Here's how the part is built. I have some questions about the finished solid (model axes, mm). A direction names the side the tool comes from. Give positions to 0.01 mm unless a question says otherwise; leave off trailing zeros. Write each loop counter-clockwise with the first axis right and the second up, starting at its lowest first coordinate (ties: lowest second). Pieces come first, ordered by that corner, then holes. Notation, with made-up numbers: M -15,-9 L 29,-9 A31 cw 29,24 Z; hole C -10.75,83 d10. An arc over 180 degrees is marked long. Answer as CSV lines item,"result". Start each with the question number.
Q1. If I drill on line 1 along X through (y, z) = (117, 0); line 2 along Z through (x, y) = (0, 81.5); line 3 along X through (y, z) = (85.5, -45), over which ranges is the centre line in solid material (lowest first)?
Q2. Suppose I cut it at D-D (z = 88). Write out the boundary of the cut face in (x, y) (1 decimal).
Q3. Thinking about a two-plate mould opening in Z: for faces 4 (the cylindrical face through (-4.62, 4.7, 144.39)), 5 (the flat face through (-1, 0, 123)), 6 (the cylindrical face through (122.834, 4.696, -50.878)), which applies, +Z half, -Z half, draft (parallel to the pull), parting line (faces both ways), or undercut?
Q4. Suppose I cut it at B-B (x = 44). Write out the boundary of the cut face in (y, z) (1 decimal).
Q5. Suppose I cut it at A-A (z = 0). Write out the boundary of the cut face in (x, y) (1 decimal).
Q6. Suppose I cut it at C-C (x = 83.5). Write out the boundary of the cut face in (y, z) (1 decimal), then the cut area to 3 significant figures.
Q7. On a 3-axis mill with a long thin cutter (end or side, diameter ignored), from which of +Z, -Z, +X, -X, +Y, -Y can I reach the whole of each face in a straight line? I mean faces 1 (the flat face through (-1, 9.525, 132)), 2 (the cylindrical face through (3.44, 55.567, 121.395)), 3 (the flat face through (-109.22, 43, -64)). Say none if no direction works.
Q8. For pin 1 (1.5 mm diameter, centred on y = 102.5, z = -12, fed in from +X); pin 2 (12 mm diameter, centred on x = 30, z = -86.5, fed in from -Y); pin 3 (5.5 mm diameter, centred on x = 126.13, z = -52.25, fed in from -Y); pin 4 (5 mm diameter, centred on y = 37.5, z = 82, fed in from +X), each with a flat end and sliding along its axis, tell me the tip position at first contact or that it passes through.
```python
from build123d import *

# Parameters (mm, degrees)
SKETCH1_R                   = 144.4625
BOSS_EXTRUDE1_DEPTH         = 9.525
F_1_4_CLEARANCE_HOLE1_D     = 7.14248
SKETCH4_R                   = 127.79375
SKETCH4_R_2                 = 121.44375
BOSS_EXTRUDE2_DEPTH         = 112.7125
BOSS_EXTRUDE3_START         = -9.525
SKETCH5_R                   = 121.44375
BOSS_EXTRUDE3_DEPTH         = 9.525
CUT_EXTRUDE1_REACH          = 240.077
SKETCH6_R                   = 121.44375
CUT_EXTRUDE2_REACH          = 240.077
SKETCH7_R                   = 51.59375
SKETCH10_W                  = 218.44
SKETCH10_H                  = 91.362820019
CUT_EXTRUDE3_DEPTH          = 112.7125
TAP_DRILL_FOR_1_4_20_TAP1_D = 5.1054


with BuildPart() as part:
    # Sketch1 → Boss-Extrude1 (new body)
    with BuildSketch(Plane(origin=(0, 0, 0), x_dir=(1, 0, 0), z_dir=(0, 1, 0))):
        with Locations(Location((0, 0, 0), (0, 0, 90))):
            Circle(SKETCH1_R)
    extrude(amount=BOSS_EXTRUDE1_DEPTH)

    # 1/4 Clearance Hole1 (through all)
    with Locations(Plane(origin=(0, 9.525, 0), x_dir=(1, 0, 0), z_dir=(0, 1, 0))):
        with Locations((0, 136.525), (-52.245855604, 126.132653176), (52.245855604, 126.132653176), (126.132653176, 52.245855604), (126.132653176, -52.245855604), (52.245855604, -126.132653176), (-52.245855604, -126.132653176), (-126.132653176, -52.245855604), (-126.132653176, 52.245855604)):
            Hole(F_1_4_CLEARANCE_HOLE1_D / 2)

    # Sketch4 → Boss-Extrude2 (add)
    with BuildSketch(Plane(origin=(0, 9.525, 0), x_dir=(1, 0, 0), z_dir=(0, 1, 0))):
        with Locations(Location((0, 0, 0), (0, 0, 90))):
            Circle(SKETCH4_R)
        with Locations(Location((0, 0, 0), (0, 0, 90))):
            Circle(SKETCH4_R_2, mode=Mode.SUBTRACT)
    extrude(amount=BOSS_EXTRUDE2_DEPTH)

    # Sketch5 → Boss-Extrude3 (add)
    with BuildSketch(Plane(origin=(0, 122.2375, 0), x_dir=(1, 0, 0), z_dir=(0, 1, 0)).offset(BOSS_EXTRUDE3_START)):
        with Locations(Location((0, 0, 0), (0, 0, 90))):
            Circle(SKETCH5_R)
    extrude(amount=BOSS_EXTRUDE3_DEPTH)

    # Sketch6 → Cut-Extrude1 (cut, up to next)
    with BuildSketch(Plane.XZ, mode=Mode.PRIVATE) as cut_extrude1_sk1:
        with Locations(Location((0, 0, 0), (0, 0, 270))):
            Circle(SKETCH6_R)
    cut_extrude1_tool1 = extrude(cut_extrude1_sk1.sketch, amount=-CUT_EXTRUDE1_REACH, mode=Mode.PRIVATE) & part.part
    add(cut_extrude1_tool1.solids().sort_by_distance((0, 0, 0))[0], mode=Mode.SUBTRACT)

    # Sketch7 → Cut-Extrude2 (cut, up to next)
    with BuildSketch(Plane(origin=(0, 122.2375, 0), x_dir=(1, 0, 0), z_dir=(0, 1, 0)), mode=Mode.PRIVATE) as cut_extrude2_sk1:
        with Locations(Location((0, 0, 0), (0, 0, 270))):
            Circle(SKETCH7_R)
    cut_extrude2_tool1 = extrude(cut_extrude2_sk1.sketch, amount=-CUT_EXTRUDE2_REACH, mode=Mode.PRIVATE) & part.part
    add(cut_extrude2_tool1.solids().sort_by_distance((0, 122.2375, 0))[0], mode=Mode.SUBTRACT)

    # Sketch10 → Cut-Extrude3 (cut)
    with BuildSketch(Plane(origin=(0, 0, 0), x_dir=(1, 0, 0), z_dir=(0, 1, 0))):
        with Locations((0, 98.781089991)):
            Rectangle(SKETCH10_W, SKETCH10_H)
    extrude(amount=CUT_EXTRUDE3_DEPTH, mode=Mode.SUBTRACT)

    # Tap Drill for 1/4-20 Tap1 (through all)
    with Locations(Plane(origin=(0, 122.2375, 0), x_dir=(1, 0, 0), z_dir=(0, 1, 0))):
        with Locations((93.487442339, -53.975), (0, -107.95), (-93.487442339, -53.975), (-93.487442339, 53.975), (0, 107.95), (93.487442339, 53.975)):
            Hole(TAP_DRILL_FOR_1_4_20_TAP1_D / 2)


solid = part.part
```
Resolved:
1,line 1,"-127.79 to -51.59, 51.59 to 127.79"
1,line 2,"121.44 to 127.79"
1,line 3,"-119.61 to -112.8, 112.8 to 119.61"
2,outline,"M -114.6,0 L -83.7,0 L -83.7,112.7 L 83.7,112.7 L 83.7,0 L 114.6,0 L 114.6,9.5 L 92.7,9.5 L 92.7,122.2 L -92.7,122.2 L -92.7,9.5 L -114.6,9.5 Z"
3,face 4,"parting line"
3,face 5,"draft"
3,face 6,"undercut"
4,outline,"M 0,113.2 L 112.7,113.2 L 112.7,26.9 L 122.2,26.9 L 122.2,120 L 9.5,120 L 9.5,137.6 L 0,137.6 Z; M 112.7,-120 L 122.2,-120 L 122.2,-26.9 L 112.7,-26.9 Z"
5,outline,"M -144.5,0 L -121.4,0 L -121.4,112.7 L -51.6,112.7 L -51.6,122.2 L -127.8,122.2 L -127.8,9.5 L -144.5,9.5 Z; M 51.6,112.7 L 121.4,112.7 L 121.4,0 L 144.5,0 L 144.5,9.5 L 127.8,9.5 L 127.8,122.2 L 51.6,122.2 Z"
6,outline,"M 0,88.2 L 112.7,88.2 L 112.7,-96.7 L 122.2,-96.7 L 122.2,96.7 L 9.5,96.7 L 9.5,117.9 L 0,117.9 Z"
6,area,"3,010 mm^2"
7,face 1,"+Y"
7,face 2,"-Y"
7,face 3,"-Z, -Y"
8,pin 1,"x = 127.3"
8,pin 2,"y = 112.71"
8,pin 3,"through"
8,pin 4,"x = 100.05"
